Job drawing, mm, ordinate dimensions from the low corner. One solid piece. A direction names the side the tool comes from. Give positions to 0.01 mm unless a question says otherwise; leave off trailing zeros. Loops run counter-clockwise (first coordinate to the right, second up) from the corner with the lowest first, then second, coordinate; pieces in that order, holes last. Notation, with made-up numbers: (-26.75, -3.5) -> (24.25, -3.5) arc R34 cw to (24.25, 27.5) -> close; hole circle Ø1 at (-34.75, -28.5). An arc over 180 degrees is marked (long way). Use one line per item in the form item = value.
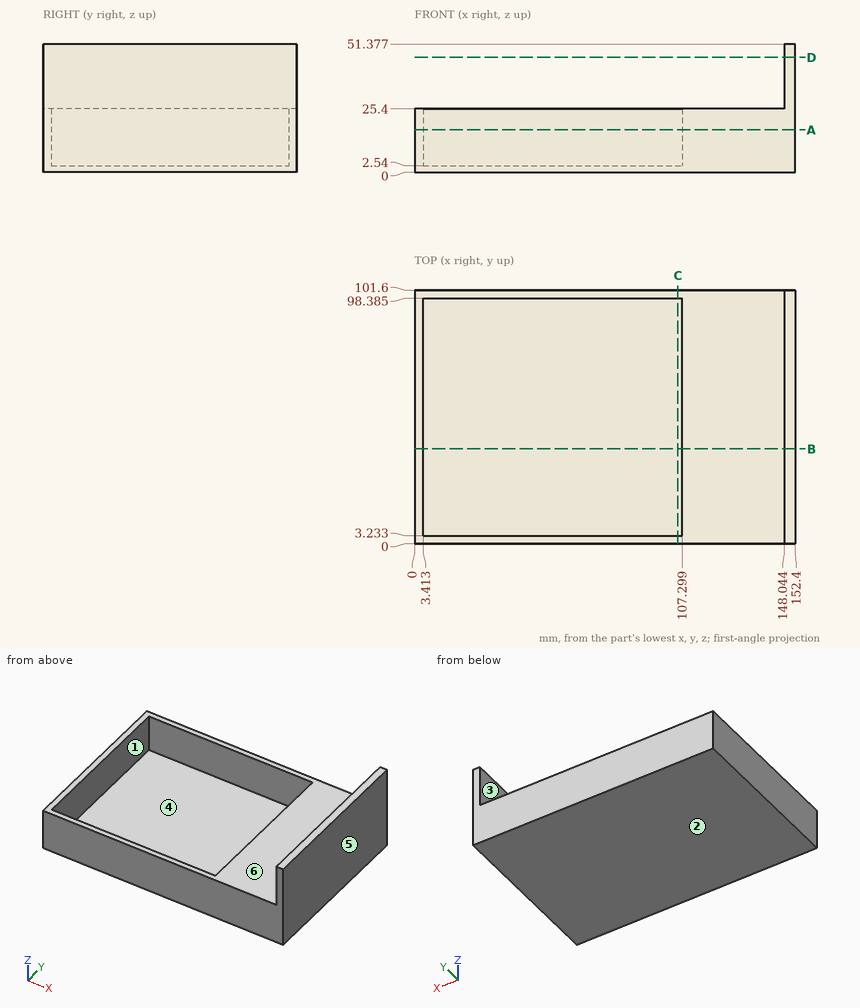
1. Cut at D-D, the plane z = 46. Write the cut outline in (x, y).
Result sheet:
outline = (148.04, 0) -> (152.4, 0) -> (152.4, 101.6) -> (148.04, 101.6) -> close
2. Drill centre lines: line 1 (X direction, y = 17.5, z = 7); line 2 (Y direction, x = 38.5, z = 22) (1 decimal); line 3 (X direction, y = 41, z = 25.5). Where is each one in solid material? Low to high.
Result sheet:
line_1 = 0 to 3.41, 107.3 to 152.4
line_2 = 0 to 3.2, 98.4 to 101.6
line_3 = 148.04 to 152.4
3. Cut at A-A, the plane z = 17. Write the cut outline in (x, y) (1 decimal).
Result sheet:
outline = (0, 0) -> (152.4, 0) -> (152.4, 101.6) -> (0, 101.6) -> close; hole (3.4, 3.2) -> (107.3, 3.2) -> (107.3, 98.4) -> (3.4, 98.4) -> close
4. Tool access for the marked faces 1, 2 and 3: list every direction of +Z, -Z, +X, -X, +Y, -Y with a clear straight run to the whole face (end or side of a thin tool).
Result sheet:
face_1 = +Z
face_2 = -Z, +X, -X, +Y, -Y
face_3 = +Z, -X, +Y, -Y
5. Mould opens along X. For the marked faces 4, 5 and 6 say: pulls with the +X half, pulls with the -X half, needs draft (parallel to the pull), parting line crosses it, or undercut.
Result sheet:
face_4 = undercut
face_5 = pulls with the +X half
face_6 = needs draft
6. Cut at B-B, the plane y = 38. Write the cut outline in (x, z).
Result sheet:
outline = (0, 0) -> (152.4, 0) -> (152.4, 51.38) -> (148.04, 51.38) -> (148.04, 25.4) -> (107.3, 25.4) -> (107.3, 2.54) -> (3.41, 2.54) -> (3.41, 25.4) -> (0, 25.4) -> close
7. Drop a flat-ended pin along its axis: P1, Ø2, axis at x = 22.5, y = 77.5, coming from the +Z side. Give the stop position or say it passes through.
Result sheet:
P1 = 2.54
8. Cut at C-C, the plane x = 105.5. Write the cut outline in (y, z) (1 decimal).
Result sheet:
outline = (0, 0) -> (101.6, 0) -> (101.6, 25.4) -> (98.4, 25.4) -> (98.4, 2.5) -> (3.2, 2.5) -> (3.2, 25.4) -> (0, 25.4) -> close
